Source: three-view drawing plus pictorial views. Frame: mm from the lowest corner of the part. A direction names the side the tool comes from. Give positions to 0.01 mm unless a question says otherwise; leave off trailing zeros. Loops run counter-clockwise (first coordinate to the right, second up) from the corner with the lowest first, then second, coordinate; pieces in that order, holes last. Notation, with made-up numbers: (75, 14.25) -> (122, 14.25) arc R33 ccw to (122, 50.25) -> close; hole circle Ø6 at (-30.5, 75). An arc over 180 degrees is marked (long way). Answer as a JSON object with one key per item and string values. Group by question number.
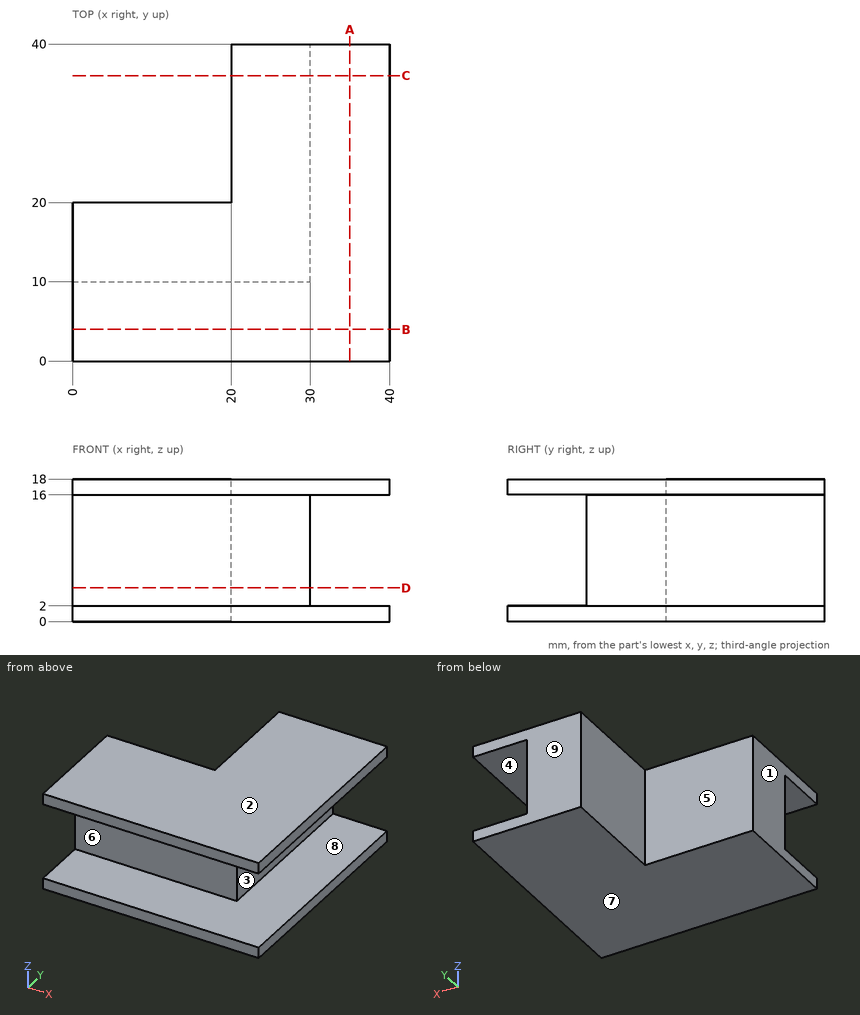
Q1. Section C-C on y = 36. Return the cut outline in (x, z).
Q2. Section D-D on z = 4.25. Return the cut outline in (x, y), then the cut area to 3 significant figures.
Q3. Pin query (flat end, axial travel): pin 1 Ø9 at (x, z) = (6.5, 5.5) entering from +Y; pin 2 Ø12 at (x, y) = (12.5, 28.5) entering from -Z; pin 3 Ø1.5 at (x, y) = (21.5, 35) entering from -Z; pin 4 Ø1 at (x, z) = (23.5, 7.5) entering from -Y. Return the tip coordinate at first contact, or that it passes through.
Q4. Set-up query: the marked faces 5, 6, 7, 8 and 9. Return all of +Z, -Z, +X, -X, +Y, -Y with unobstructed straight access to the full face (end or side cutting, diameter ignored); none if empty.
Q5. Ray query, probe 1 along Z at (x, y) = (10, 5); probe 2 along X at (y, z) = (28, 14); probe 3 along Y at (x, z) = (2, 10.5). Return the intervals inside material, ascending.
Q6. Section A-A on x = 35. Return the cut outline in (y, z), then the cut area to 3 significant figures.
Q7. Pull-direction query (Z, two-part tool) for the marked faces 1, 2, 3 and 4; classes: +Z half, -Z half, draft (parallel to the pull), parting line (faces both ways), or undercut.
Numbers:
{
 "1": {"outline": "(20, 0) -> (40, 0) -> (40, 2) -> (30, 2) -> (30, 16) -> (40, 16) -> (40, 18) -> (20, 18) -> close"},
 "2": {"outline": "(0, 10) -> (30, 10) -> (30, 40) -> (20, 40) -> (20, 20) -> (0, 20) -> close", "area": "500 mm²"},
 "3": {"pin 1": "stops at y = 20", "pin 2": "passes through", "pin 3": "stops at z = 0", "pin 4": "stops at y = 10"},
 "4": {"face 5": "+Z, -Z, -X, +Y", "face 6": "+X, -X, -Y", "face 7": "-Z, +X, -X, +Y, -Y", "face 8": "+X, -Y", "face 9": "+Z, -Z, +X, -X, +Y"},
 "5": {"probe 1": "z = 0 to 2, 16 to 18", "probe 2": "x = 20 to 30", "probe 3": "y = 10 to 20"},
 "6": {"outline": "(0, 0) -> (40, 0) -> (40, 2) -> (0, 2) -> close; (0, 16) -> (40, 16) -> (40, 18) -> (0, 18) -> close", "area": "160 mm²"},
 "7": {"face 1": "draft", "face 2": "+Z half", "face 3": "undercut", "face 4": "undercut"}
}
